Drawing for the job (mm, zero at the part's lowest x, y, z). Give positions to 0.01 mm unless a question says otherwise; leave off trailing zeros. Write each loop counter-clockwise with the first axis right and the second up, starting at its lowest first coordinate (ties: lowest second). Pieces come first, ordered by that corner, then holes. Notation, with made-up numbers: M 29,31.5 L 85,31.5 A22 ccw 85,58.5 Z; hole C 56,72 d6. An arc over 180 degrees is marked long. Answer as a JSON object with one key per item and string values. Group by question number.
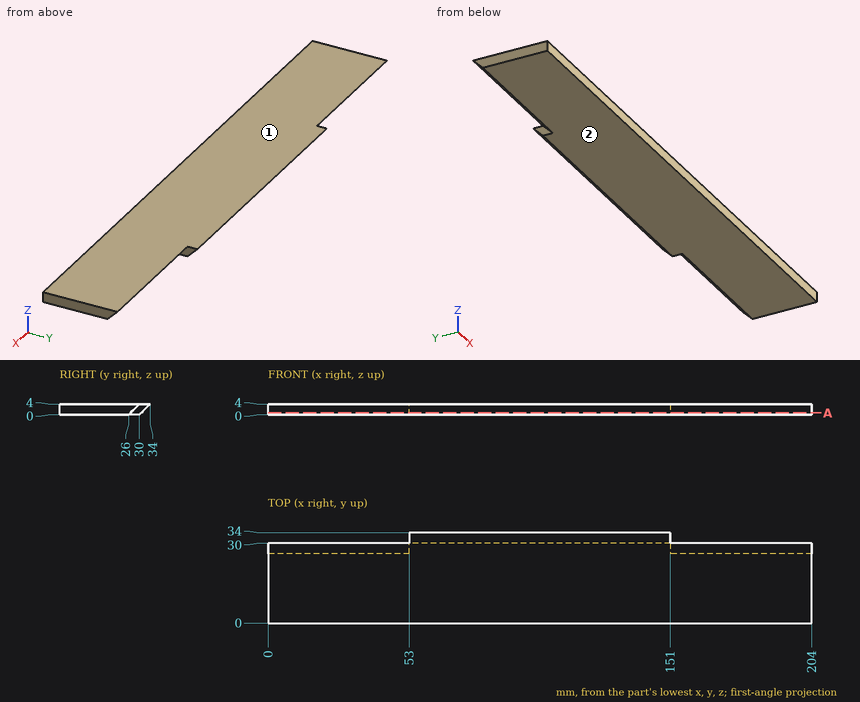
Q1. Two-plate mould, pull along Z, no slides. Class the marked faces 1 and 2: +Z half, -Z half, draft (parallel to the pull), parting line (faces both ways), or undercut.
Q2. Drop flat-ended pins along their axis: P1, Ø1.2, axis at y = 29.5, z = 2, coming from the -X side; P2, Ø1, axis at x = 142, z = 1, coming from the +Y side. Give the stop position or say it passes through.
Q3. Slice it at A-A, the plane z = 0.7. Write the cut outline in (x, y).
Q4. Wall check: L1, parallel to X at y = 32, z = 3.05; L2, parallel to Y at x = 146, z = 0.75; L3, parallel to Y at x = 20.5, z = 2.55. Give the ranges that are in metal, low to high.
Solved:
{
 "1": {"face 1": "+Z half", "face 2": "-Z half"},
 "2": {"P1": "stops at x = 53", "P2": "stops at y = 31.5"},
 "3": {"outline": "M 0,0 L 204,0 L 204,26.7 L 151,26.7 L 151,30.7 L 53,30.7 L 53,26.7 L 0,26.7 Z"},
 "4": {"L1": "x = 53 to 151", "L2": "y = 0 to 30.75", "L3": "y = 0 to 28.55"}
}
